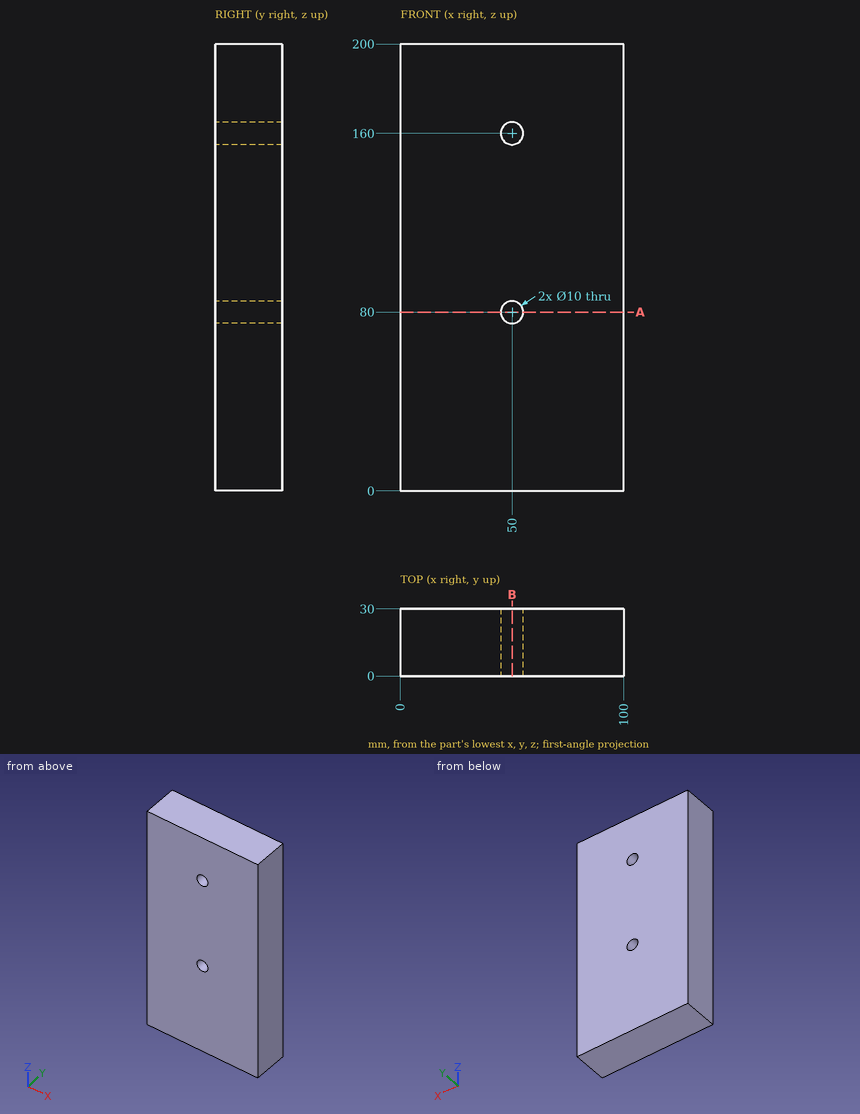
Input: dimensioned drawing with shaded views. Units: mm. Origin: part minimum x, y, z. Give positions to 0.01 mm unless a question says otherwise; leave off trailing zeros. Write each loop counter-clockwise with the first axis right and the second up, starting at its lowest first coordinate (ties: lowest second). Pieces come first, ordered by that corner, then holes.
1. Line query: probe 1 along Z at (x, y) = (50, 21.75); probe 2 along X at (y, z) = (22.25, 160); probe 3 along X at (y, z) = (16.25, 79). Output: solid intervals per line, ascending.
2. Section query B-B, the plane x = 50. Return loops of the section in (y, z), then the cut area to 3 significant figures.
3. Section query A-A, the plane z = 80. Return loops of the section in (x, y).
Computed:
1. probe 1: z = 0 to 75, 85 to 155, 165 to 200
1. probe 2: x = 0 to 45, 55 to 100
1. probe 3: x = 0 to 45.1, 54.9 to 100
2. outline: (0, 0) - (30, 0) - (30, 75) - (0, 75) - close; (0, 85) - (30, 85) - (30, 155) - (0, 155) - close; (0, 165) - (30, 165) - (30, 200) - (0, 200) - close
2. area: 5,400 mm2
3. outline: (0, 0) - (45, 0) - (45, 30) - (0, 30) - close; (55, 0) - (100, 0) - (100, 30) - (55, 30) - close
